Source: CAD feature listing. Evaluate the final solid. Frame: model axes, mm. A direction names the side the tool comes from. Coordinates: 2 decimals unless noted, no trailing zeros. Order: outer loops, then holes, each group sorted by start corner. A loop starts at its lowest first (then second) coordinate and runs counter-clockwise, first axis right, second up.
```python
from build123d import *

# Parameters (mm, degrees)
CROQUIS1_W              = 6.7
CROQUIS1_H              = 3.7
SALIENTE_EXTRUIR1_DEPTH = 1.3
SALIENTE_EXTRUIR1_TAPER = 5
CROQUIS1_2_W            = 6.7
CROQUIS1_2_H            = 3.7
SALIENTE_EXTRUIR2_DEPTH = 0.4
SALIENTE_EXTRUIR2_DRAFT = -5
BARRER1_START           = -0.42
BARRER1_DEPTH           = 0.84
MATRIZL1_COUNT          = 2
MATRIZL1_PITCH          = 2.3
MATRIZL2_COUNT          = 2
MATRIZL2_PITCH          = 2.3
BARRER2_START           = -1.55
BARRER2_DEPTH           = 3.1


# Read off the part's stored shape, not the designer's step: Barrer1, Barrer2
with BuildPart() as part:
    # Croquis1 → Saliente-Extruir1 (new body)
    with BuildSketch(Plane(origin=(0, 0, 0), x_dir=(1, 0, 0), z_dir=(0, 1, 0))):
        Rectangle(CROQUIS1_W, CROQUIS1_H)
    extrude(amount=SALIENTE_EXTRUIR1_DEPTH, taper=SALIENTE_EXTRUIR1_TAPER)


with BuildPart() as saliente_extruir2_tool:
    # Croquis1<2> → Saliente-Extruir2 (with draft: the straight prism first)
    with BuildSketch(Plane(origin=(0, 0, 0), x_dir=(1, 0, 0), z_dir=(0, 1, 0))):
        Rectangle(CROQUIS1_2_W, CROQUIS1_2_H)
    extrude(amount=-SALIENTE_EXTRUIR2_DEPTH)
    # Saliente-Extruir2: the draft: its side faces are tilted about the plane it starts from
    saliente_extruir2_sides = [saliente_extruir2_tool.faces().sort_by_distance(p)[0] for p in [
        (-3.35, -0.2, 0),
        (0, -0.2, 1.85),
        (3.35, -0.2, 0),
        (0, -0.2, -1.85),
    ]]
    draft(saliente_extruir2_sides, Plane(origin=(0, 0, 0), x_dir=(1, 0, 0), z_dir=(0, 1, 0)), SALIENTE_EXTRUIR2_DRAFT)


with BuildPart() as part_1:
    add(part.part)

    # Saliente-Extruir2: add saliente_extruir2_tool
    add(saliente_extruir2_tool.part)

    # Barrer1 outline → Barrer1 (add)
    with BuildSketch(Plane.YZ.offset(BARRER1_START)):
        with BuildLine():
            Line((0.35, -2.098236587), (0.35, -1.819378968))
            Line((0.35, -1.819378968), (0, -1.85))
            Line((0, -1.85), (0, -2.098236587))
            ThreePointArc((0, -2.098236587), (-0.002534971, -2.109205747), (-0.009625798, -2.117950387))
            Line((-0.009625798, -2.117950387), (-0.151773886, -2.228807417))
            ThreePointArc((-0.151773886, -2.228807417), (-0.24251362, -2.331233787), (-0.290463768, -2.459396356))
            Line((-0.290463768, -2.459396356), (-0.492341357, -3.604301053))
            Line((-0.492341357, -3.604301053), (-0.147658643, -3.665077915))
            Line((-0.147658643, -3.665077915), (0.054218945, -2.520173218))
            ThreePointArc((0.054218945, -2.520173218), (0.057415622, -2.511629047), (0.063464937, -2.504800622))
            Line((0.063464937, -2.504800622), (0.205613025, -2.393943592))
            ThreePointArc((0.205613025, -2.393943592), (0.311975433, -2.262773993), (0.35, -2.098236587))
        make_face()
    barrer1 = extrude(amount=BARRER1_DEPTH)

    # MatrizL1: Barrer1 ×2
    with Locations(*[(-i * MATRIZL1_PITCH, 0, 0) for i in range(1, MATRIZL1_COUNT)]):
        add(barrer1)

    # MatrizL2: Barrer1 ×2
    with Locations(*[(i * MATRIZL2_PITCH, 0, 0) for i in range(1, MATRIZL2_COUNT)]):
        add(barrer1)

    # Barrer2 outline → Barrer2 (add)
    with BuildSketch(Plane.YZ.offset(BARRER2_START)):
        with BuildLine():
            Line((0.35, 1.819378968), (0.35, 2.094689484))
            ThreePointArc((0.35, 2.094689484), (0.314483055, 2.253988747), (0.214659972, 2.383112954))
            Line((0.214659972, 2.383112954), (0.073760247, 2.500190888))
            ThreePointArc((0.073760247, 2.500190888), (0.068117087, 2.506867054), (0.065117385, 2.515077915))
            Line((0.065117385, 2.515077915), (-0.137658643, 3.665077915))
            Line((-0.137658643, 3.665077915), (-0.482341357, 3.604301053))
            Line((-0.482341357, 3.604301053), (-0.279565329, 2.454301053))
            ThreePointArc((-0.279565329, 2.454301053), (-0.234569796, 2.33113814), (-0.149922393, 2.23099565))
            Line((-0.149922393, 2.23099565), (-0.009022669, 2.113917715))
            ThreePointArc((-0.009022669, 2.113917715), (-0.002367796, 2.105309435), (0, 2.094689484))
            Line((0, 2.094689484), (0, 1.85))
            Line((0, 1.85), (0.35, 1.819378968))
        make_face()
    extrude(amount=BARRER2_DEPTH)


solid = part_1.part
```
1. Section query A-A on z = -2. Return loops of the section in (x, y), plus the area to 3 significant figures.
Findings:
outline: (-2.72, 0) - (-1.88, 0) - (-1.88, 0.35) - (-2.72, 0.35) - close; (-0.42, 0) - (0.42, 0) - (0.42, 0.35) - (-0.42, 0.35) - close; (1.88, 0) - (2.72, 0) - (2.72, 0.35) - (1.88, 0.35) - close
area: 0.882 mm2
2. Access query for faces 5 (the face through (2.29, -0.39, -3.02)), 6 (the face through (-0.01, -0.05, -3.1)). Directions: +Z, -Z, +X, -X, +Y, -Y. A direction counts if a zero-diameter tool reaches every point of the face in a straight line with its end or side. Return the directions, or none.
Findings:
face 5: +X, -X, -Y
face 6: -Z, +X, -X, +Y
3. Draft query along Z for faces 1 (the face through (-0.022, -0.382, 3.037)), 2 (the face through (1.88, -0.17, -2.73)), 3 (the face through (-0.022, -0.035, 3.082)), 4 (the face through (2.29, -0.05, -3.1)). Return one class per face: released by +Z, released by -Z, zero draft, split by the parting line, or undercut.
Findings:
face 1: undercut
face 2: zero draft
face 3: released by +Z
face 4: released by -Z
4. Ray query, line 1 (X direction, y = -0.3, z = -3.25); line 2 (Y direction, x = -2.75, z = -1.25); line 3 (X direction, y = 1.2, z = -0.5). Return the intervals inside material, ascending.
Findings:
line 1: x = -2.72 to -1.88, -0.42 to 0.42, 1.88 to 2.72
line 2: y = -0.4 to 1.3
line 3: x = -3.25 to 3.25
5. Pin query (flat end, axial travel): P1, Ø4, axis at x = 0.5, z = 0, coming from the -Y side; P2, Ø0.9, axis at y = 0, z = -3, coming from the -X side; P3, Ø0.7, axis at y = -0.5, z = 2.5, coming from the +X side. Return the tip coordinate at first contact, or that it passes through.
Findings:
P1: stops at y = -0.4
P2: stops at x = -2.72
P3: stops at x = 1.55
